Here's how the part is built. I have some questions about the finished solid (model axes, mm). A direction names the side the tool comes from. Round coordinates to 2 decimals unless told otherwise and drop trailing zeros. Loops run counter-clockwise (first coordinate to the right, second up) from the corner with the lowest first, then second, coordinate; pieces in that order, holes last. Notation, with made-up numbers: M 17,61.25 L 72,61.25 A23 cw 72,87.25 Z; hole C -9.5,71.5 d5. An arc over 180 degrees is marked long. Answer as CSV lines item,"result".
```python
from build123d import *

# Parameters (mm, degrees)
SKETCH1_W           = 20
SKETCH1_H           = 3
SKETCH1_W_2         = 1.5
SKETCH1_H_2         = 1.5
BOSS_EXTRUDE1_DEPTH = 1
SKETCH1_3_W         = 1.5
SKETCH1_3_H         = 1.5
BOSS_EXTRUDE2_DEPTH = 3


with BuildPart() as part:
    # Sketch1 → Boss-Extrude1 (new body)
    with BuildSketch(Plane(origin=(0, 0, 0), x_dir=(1, 0, 0), z_dir=(0, 1, 0))):
        with Locations((10, 1.5)):
            Rectangle(SKETCH1_W, SKETCH1_H)
        with Locations((2.25, 1.5)):
            Rectangle(SKETCH1_W_2, SKETCH1_H_2, mode=Mode.SUBTRACT)
        with Locations((17.75, 1.5)):
            Rectangle(SKETCH1_W_2, SKETCH1_H_2, mode=Mode.SUBTRACT)
    extrude(amount=BOSS_EXTRUDE1_DEPTH)

    # Sketch1<3> → Boss-Extrude2 (add)
    with BuildSketch(Plane(origin=(0, 0, 0), x_dir=(1, 0, 0), z_dir=(0, 1, 0))):
        with Locations((2.25, 1.5)):
            Rectangle(SKETCH1_3_W, SKETCH1_3_H)
        with Locations((17.75, 1.5)):
            Rectangle(SKETCH1_3_W, SKETCH1_3_H)
    extrude(amount=BOSS_EXTRUDE2_DEPTH)


solid = part.part
```
1. Which directions (+Z, -Z, +X, -X, +Y, -Y) give clear straight access to the entire face, cutting with the end or side of a thin tool? Please do faces 4 (the flat face through (2, 2, -2.25)), 5 (the flat face through (18.5, 2, -1)), 6 (the flat face through (3, 2, -1)), 7 (the flat face through (1.5, 2, -1)), 8 (the flat face through (2, 2, -0.75)).
Evaluation:
face 4,"-Z, +X, -X, +Y"
face 5,"+Z, -Z, +X, +Y"
face 6,"+Z, -Z, +Y"
face 7,"+Z, -Z, -X, +Y"
face 8,"+Z, +X, -X, +Y"
2. I want a section at A-A, the plane y = 1.95. Please give me the cut outline in (x, z), and give its area (3 significant figures).
Evaluation:
outline,"M 1.5,-2.25 L 3,-2.25 L 3,-0.75 L 1.5,-0.75 Z; M 17,-2.25 L 18.5,-2.25 L 18.5,-0.75 L 17,-0.75 Z"
area,"4.50 mm²"
3. For P1, Ø0.8, axis at x = 2.5, y = 1.5, coming from the +Z side; P2, Ø1.6, axis at y = 2, z = -1.5, coming from the -X side; P3, Ø1.2, axis at x = 17.5, y = 1.5, coming from the +Z side; P4, Ø0.8, axis at y = 1.5, z = -1.5, coming from the +X side, each with a flat end and sliding along its axis, tell me the tip position at first contact or that it passes through.
Evaluation:
P1,"stops at z = -0.75"
P2,"stops at x = 1.5"
P3,"stops at z = 0"
P4,"stops at x = 18.5"
4. I want a section at C-C, the plane x = 7.75. Please give me the cut outline in (y, z), and give its area (3 significant figures).
Evaluation:
outline,"M 0,-3 L 1,-3 L 1,0 L 0,0 Z"
area,"3.00 mm²"
5. If I drill on line 1 (X direction, y = 2, z = -2.15); line 2 (Y direction, x = 5.5, z = -0.3), over which ranges is the centre line in solid material (lowest first)? Write a range as [from, to].
Evaluation:
line 1,"x = [1.5, 3], [17, 18.5]"
line 2,"y = [0, 1]"
6. We'd pull the mould along X, two halves only. Please class faces 1 (the flat face through (18, 2, -0.75)), 2 (the flat face through (20, 0.5, -1.5)), 3 (the flat face through (17, 2, -1)): pulls with the +X half, pulls with the -X half, needs draft (parallel to the pull), parting line crosses it, or undercut.
Evaluation:
face 1,"needs draft"
face 2,"pulls with the +X half"
face 3,"undercut"
7. I want a section at B-B, the plane z = -1. Please give me the cut outline in (x, y).
Evaluation:
outline,"M 0,0 L 20,0 L 20,1 L 18.5,1 L 18.5,3 L 17,3 L 17,1 L 3,1 L 3,3 L 1.5,3 L 1.5,1 L 0,1 Z"
